For this review, take the finished solid that the model builds, in its own axes (mm). Face numbers are marked on the shaded views. Coordinates: 2 decimals unless noted, no trailing zeros. Write each loop counter-clockwise with the first axis right and the second up, starting at its lowest first coordinate (ties: lowest second). Pieces come first, ordered by that corner, then holes. Notation, with made-up numbers: (19, 16.25) - (42, 16.25) arc R25 ccw to (42, 47.25) - close; hole circle Ø4 at (-3.75, 1). An arc over 180 degrees is marked (long way). Use one line per item in the form item = value. Start each with the question number.
1) Insertion check: P1, Ø10, axis at x = 134, z = 442, coming from the +Y side; P2, Ø6.5, axis at x = 714.5, z = 757, coming from the +Y side; P3, Ø4.5, axis at x = 1376.75, z = 1115.5, coming from the +Y side. Each pin has a flat end and moves straight along its axis. Give the tip position at first contact, or say it passes through.
2) We need section D-D (z = 702.5). Give the boundary of the cut face in (x, y).
3) Mouldability with a two-part tool opening along X and no side actions: class the marked faces 1 and 2 as pulls with the +X half, pulls with the -X half, needs draft (parallel to the pull), parting line crosses it, or undercut.
4) We need section A-A (y = 438). Give the boundary of the cut face in (x, z), plus the area to 3 significant figures.
5) We need section B-B (x = 928). Give the boundary of the cut face in (y, z) (3 decimals).
6) For L1, parallel to X at y = 8.25, z = 1015.5; L2, parallel to Z at x = 851.5, y = 57; L3, parallel to Z at x = 1376.75, y = 8.25, list the stretches that pass through material, from the lowest coordinate up. Write a range as from..to.
7) We need section C-C (z = 227.5). Give the boundary of the cut face in (x, y).
```python
from build123d import *

# Parameters (mm, degrees)
F0_W      = 1430
F0_H      = 1730
F0_W_2    = 50
F0_H_2    = 5
F0_W_3    = 1077.78
F0_H_3    = 608
F1_DEPTH  = 12.7
F2_W      = 664.2
F2_H      = 12.7
F2_W_2    = 50.8
F2_H_2    = 50.8
F3_DEPTH  = 76.2
F4_W      = 1328.4
F4_H      = 12.7
F5_DEPTH  = 76.2
F6_W      = 1379.2
F6_H      = 120.65
F6_W_2    = 1328.4
F6_H_2    = 107.95
F7_DEPTH  = 9.525
F8_W      = 400
F8_H      = 76.2
F9_DEPTH  = 50.8
F11_DEPTH = 50.8
F12_R     = 12.7
F12_W     = 50
F12_H     = 5
F13_DEPTH = 12.7
F15_W     = 400
F15_H     = 76.2
F16_DEPTH = 50.8
F18_DEPTH = 50.8
F19_R     = 1.75
F20_DEPTH = 12.701
F14_R     = 12.7
F21_DEPTH = 50.801
F22_W     = 304.8
F22_H     = 12.7
F23_DEPTH = 177.8
F25_DEPTH = 12.7


with BuildPart() as f1:
    # F0 (on Front) → F1 (new body)
    with BuildSketch(Plane.XZ):
        with Locations((715, 865)):
            Rectangle(F0_W, F0_H)
        with Locations((715, 891.7)):
            Rectangle(F0_W_2, F0_H_2, mode=Mode.SUBTRACT)
        with Locations((715, 1238.2)):
            Rectangle(F0_W_3, F0_H_3, mode=Mode.SUBTRACT)
    extrude(amount=-F1_DEPTH)

    # F2 (on face) → F3 (join)
    with BuildSketch(Plane(origin=(0, 12.7, 0), x_dir=(-1, 0, 0), z_dir=(0, 1, 0))):
        with Locations((-1047.1, 1723.65)):
            Rectangle(F2_W, F2_H)
        with Locations((-1404.6, 1723.65)):
            Rectangle(F2_W_2, F2_H)
        Polygon((-1379.2, 50.8), (-1379.2, 1717.3), (-1430, 1717.3), (-1430, 737.95), (-1430, 718.9), (-1430, 50.8), align=None)
        with Locations((-382.9, 1723.65)):
            Rectangle(F2_W, F2_H)
        with Locations((-1047.1, 25.4)):
            Rectangle(F2_W, F2_H_2)
        with Locations((-1404.6, 25.4)):
            Rectangle(F2_W_2, F2_H_2)
        with Locations((-25.4, 1723.65)):
            Rectangle(F2_W_2, F2_H)
        with Locations((-382.9, 25.4)):
            Rectangle(F2_W, F2_H_2)
        Polygon((0, 1717.3), (-50.8, 1717.3), (-50.8, 50.8), (0, 50.8), (0, 718.9), (0, 737.95), align=None)
        with Locations((-25.4, 25.4)):
            Rectangle(F2_W_2, F2_H_2)
    extrude(amount=F3_DEPTH)

    # F4 (on face) → F5 (join)
    with BuildSketch(Plane(origin=(0, 12.7, 0), x_dir=(-1, 0, 0), z_dir=(0, 1, 0))):
        with Locations((-715, 759.2)):
            Rectangle(F4_W, F4_H)
    extrude(amount=F5_DEPTH)

    # F6 (on face) → F7 (join)
    with BuildSketch(Plane(origin=(0, 88.9, 0), x_dir=(-1, 0, 0), z_dir=(0, 1, 0))):
        with Locations((-740.4, 1669.675)):
            Rectangle(F6_W, F6_H)
        with Locations((-715, 819.525)):
            Rectangle(F6_W_2, F6_H_2)
    extrude(amount=-F7_DEPTH)

    # F8 (on face) → F9 (join)
    with BuildSketch(Plane.YZ.offset(1430)):
        with Locations((288.9, 38.1)):
            Rectangle(F8_W, F8_H)
    extrude(amount=-F9_DEPTH)

    # F10 (on face) → F11 (join)
    with BuildSketch(Plane.YZ.offset(1430)):
        Polygon((381.1369265472, 76.2), (488.9, 76.2), (88.9, 476.2), (88.9, 368.4369265472), align=None)
    extrude(amount=-F11_DEPTH)

    # F12 (on face) → F13 (cut, through all)
    with BuildSketch(Plane.XY.offset(765.55)):
        with Locations((67.7, 42.86)):
            Circle(F12_R)
        with Locations((715, 27.5)):
            Rectangle(F12_W, F12_H)
    extrude(amount=-F13_DEPTH, mode=Mode.SUBTRACT)

    # F15 (on face) → F16 (join)
    with BuildSketch(Plane(origin=(0, 0, 0), x_dir=(0, -1, 0), z_dir=(-1, 0, 0))):
        with Locations((-288.9, 38.1)):
            Rectangle(F15_W, F15_H)
    extrude(amount=-F16_DEPTH)

    # F17 (on face) → F18 (join)
    with BuildSketch(Plane(origin=(0, 0, 0), x_dir=(0, -1, 0), z_dir=(-1, 0, 0))):
        Polygon((-88.9, 476.2), (-488.9, 76.2), (-381.1369265472, 76.2), (-88.9, 368.4369265472), align=None)
    extrude(amount=-F18_DEPTH)

    # F19 (on face) → F20 (cut, through all)
    with BuildSketch(Plane(origin=(0, 12.7, 0), x_dir=(-1, 0, 0), z_dir=(0, 1, 0))):
        with Locations((-1376.7500453753, 1406.2865250229)):
            Circle(F19_R)
        with Locations((-1376.2000453753, 1506.3180125114)):
            Circle(F19_R)
        with Locations((-1376.75, 1115.5)):
            Circle(F19_R)
        with Locations((-1376.75, 1015.5)):
            Circle(F19_R)
        with Locations((-160.41, 1448.3)):
            Circle(F19_R)
        with Locations((-160.41, 1318.3)):
            Circle(F19_R)
        with Locations((-160.41, 1168.3)):
            Circle(F19_R)
        with Locations((-160.41, 1038.3)):
            Circle(F19_R)
    extrude(amount=-F20_DEPTH, mode=Mode.SUBTRACT)

    # F14 (on face) → F21 (cut, through all)
    with BuildSketch(Plane.XY.offset(50.8)):
        with Locations((67.7, 42.86)):
            Circle(F14_R)
    extrude(amount=-F21_DEPTH, mode=Mode.SUBTRACT)

    # F22 (on face) → F23 (join)
    with BuildSketch(Plane(origin=(0, 12.7, 0), x_dir=(-1, 0, 0), z_dir=(0, 1, 0))):
        with Locations((-203.2, 441.7)):
            Rectangle(F22_W, F22_H)
    extrude(amount=F23_DEPTH)

    # F24 (on face) → F25 (join)
    with BuildSketch(Plane.YZ.offset(355.6)):
        Polygon((81.0198792071, 435.35), (63.2197438789, 435.35), (12.7, 384.8302561211), (12.7, 375.85), (12.7, 366.8697438789), align=None)
    extrude(amount=-F25_DEPTH)


solid = f1.part
```
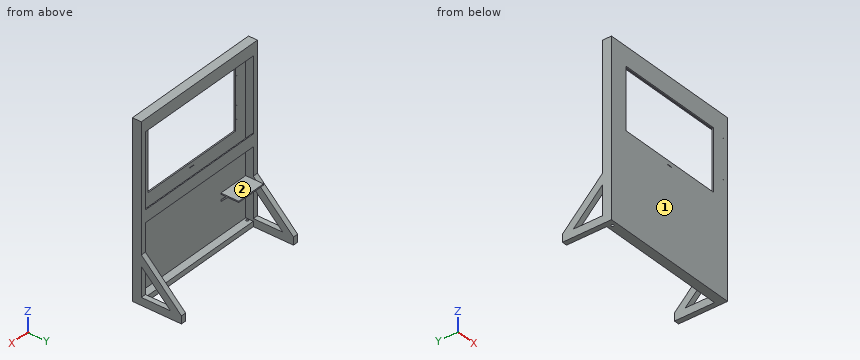
Determined:
q1.P1 = 190.5
q1.P2 = 88.9
q1.P3 = 12.7
q2.outline = (0, 0) - (1430, 0) - (1430, 88.9) - (1379.2, 88.9) - (1379.2, 12.7) - (50.8, 12.7) - (50.8, 88.9) - (0, 88.9) - close
q3.face_1 = needs draft
q3.face_2 = undercut
q4.outline = (0, 0) - (50.8, 0) - (50.8, 127.1) - (0, 127.1) - close; (1379.2, 0) - (1430, 0) - (1430, 127.1) - (1379.2, 127.1) - close
q4.area = 12,900 mm²
q5.outline = (0, 0) - (88.9, 0) - (88.9, 50.8) - (12.7, 50.8) - (12.7, 752.85) - (88.9, 752.85) - (88.9, 873.5) - (79.375, 873.5) - (79.375, 765.55) - (12.7, 765.55) - (12.7, 934.2) - (0, 934.2) - close; (0, 1542.2) - (12.7, 1542.2) - (12.7, 1717.3) - (79.375, 1717.3) - (79.375, 1609.35) - (88.9, 1609.35) - (88.9, 1730) - (0, 1730) - close
q6.L1 = 0..176.11, 1253.89..1375, 1378.5..1430
q6.L2 = 0..50.8, 752.85..765.55, 1717.3..1730
q6.L3 = 0..1013.75, 1017.25..1113.75, 1117.25..1404.54, 1408.04..1504.66, 1507.98..1730
q7.outline = (0, 0) - (1430, 0) - (1430, 88.9) - (1379.2, 88.9) - (1379.2, 12.7) - (50.8, 12.7) - (50.8, 88.9) - (0, 88.9) - close; (0, 229.84) - (50.8, 229.84) - (50.8, 337.6) - (0, 337.6) - close; (1379.2, 229.84) - (1430, 229.84) - (1430, 337.6) - (1379.2, 337.6) - close
